Work out the finished part from the listing and answer in its coordinate system (mm). A direction names the side the tool comes from. Give positions to 0.01 mm unless a question says otherwise; leave off trailing zeros. Loops run counter-clockwise (first coordinate to the right, second up) from the corner with the lowest first, then second, coordinate; pieces in that order, holes last. Notation, with made-up numbers: M 48.5,28 L 96.5,28 A14 ccw 96.5,53 Z; hole C 65,21.5 d9. An arc over 180 degrees is marked long. Use a Markdown table: item, result.
```python
from build123d import *

# Parameters (mm, degrees)
SKETCH_W        = 64
SKETCH_H        = 54
PAD_DEPTH       = 17
SKETCH001_W     = 12.371217
SKETCH001_H     = 20
POCKET_DEPTH    = 64.001
SKETCH002_W     = 32
SKETCH002_H     = 23.71851
POCKET001_DEPTH = 34.001
PAD001_DEPTH    = 24
SKETCH005_R     = 10
POCKET002_DEPTH = 64.001
SKETCH006_W     = 20
SKETCH006_H     = 14.23518
POCKET003_DEPTH = 54.001
SKETCH007_R     = 15
POCKET004_DEPTH = 48.001
SKETCH008_R     = 4
POCKET005_DEPTH = 10


with BuildPart() as pocket001:
    # Sketch → Pad (new body, symmetric)
    with BuildSketch(Plane.YZ):
        with Locations((0, 27)):
            Rectangle(SKETCH_W, SKETCH_H)
    extrude(amount=PAD_DEPTH, both=True)

    # Sketch001 → Pocket (cut, through all)
    with BuildSketch(Plane(origin=(0, -32, 0), x_dir=(0, 0, -1), z_dir=(0, -1, 0))):
        with Locations((0.185608, 0)):
            Rectangle(SKETCH001_W, SKETCH001_H)
    extrude(amount=-POCKET_DEPTH, mode=Mode.SUBTRACT)

    # Sketch002 → Pocket001 (cut, through all)
    with BuildSketch(Plane.YZ.offset(17)):
        with Locations((0, 3.140745)):
            Rectangle(SKETCH002_W, SKETCH002_H)
    extrude(amount=-POCKET001_DEPTH, mode=Mode.SUBTRACT)


with BuildPart() as pocket005:
    # Sketch004 → Pad001 (new body, symmetric)
    with BuildSketch(Plane.YZ):
        with BuildLine():
            Line((-16, 0), (-16, 15))
            Line((-16, 15), (16, 15))
            Line((16, 15), (16, 0))
            Line((16, 0), (22, 0))
            Line((22, 0), (22, 38))
            ThreePointArc((22, 38), (0, 60.000055), (-22, 38))
            Line((-22, 0), (-22, 38))
            Line((-16, 0), (-22, 0))
        make_face()
    extrude(amount=PAD001_DEPTH, both=True)

    # Fusion: union Pocket001
    add(pocket001.part)

    # Sketch005 → Pocket002 (cut, through all)
    with BuildSketch(Plane.XZ.offset(32)):
        with Locations((0, 38)):
            Circle(SKETCH005_R)
    extrude(amount=-POCKET002_DEPTH, mode=Mode.SUBTRACT)

    # Sketch006 → Pocket003 (cut, through all)
    with BuildSketch(Plane.XZ.offset(22)):
        with Locations((0, -1.11759)):
            Rectangle(SKETCH006_W, SKETCH006_H)
    extrude(amount=-POCKET003_DEPTH, mode=Mode.SUBTRACT)

    # Sketch007 → Pocket004 (cut, through all)
    with BuildSketch(Plane.YZ.offset(24)):
        with Locations((0, 38)):
            Circle(SKETCH007_R)
    extrude(amount=-POCKET004_DEPTH, mode=Mode.SUBTRACT)

    # Sketch008 → Pocket005 (cut)
    with BuildSketch(Plane.XY.offset(54)):
        with Locations((0, -23.848572)):
            Circle(SKETCH008_R)
        with Locations((0, 24.151428)):
            Circle(SKETCH008_R)
    extrude(amount=-POCKET005_DEPTH, mode=Mode.SUBTRACT)


solid = pocket005.part
```
(1) A cutting plane is placed at D-D (x = 12). Write down the section's boundary in (y, z).
Entries:
| item | result |
|---|---|
| outline | M -32,0 L -16,0 L -16,15 L 16,15 L 16,0 L 32,0 L 32,54 L 15.1,54 A22 ccw -15.1,54 L -32,54 Z; hole C 0,38 d30 |
(2) Consider probe 1 along X at (y, z) = (21, 38); probe 2 along X at (y, z) = (-26.75, 38); probe 3 along Y at (x, z) = (0, 50). Determine where each line is inside the solid, lowest interval first. Write a range as [from, to].
Entries:
| item | result |
|---|---|
| probe 1 | x = [-24, -10], [10, 24] |
| probe 2 | x = [-17, -10], [10, 17] |
| probe 3 | y = [-32, -27.85], [-19.85, -9], [9, 20.15], [28.15, 32] |
(3) Which of the six approach directions +Z, -Z, +X, -X, +Y, -Y give full straight-line access (tool end or side, diameter ignored) to faces 4 (the flat face through (4, -22, 54)), 5 (the flat face through (10, 24, 3)), 6 (the flat face through (-20, 22, 19)), 7 (the flat face through (21, -22, 19)), 8 (the cylindrical face through (-3.996, -23.673, 50.63))?
Entries:
| item | result |
|---|---|
| face 4 | +Z, +X, -X, -Y |
| face 5 | -Z, +Y, -Y |
| face 6 | +Z, -Z, -X, +Y |
| face 7 | +Z, -Z, +X, -Y |
| face 8 | +Z |
(4) A cutting plane is placed at A-A (y = 0). Write down the section's boundary in (x, z).
Entries:
| item | result |
|---|---|
| outline | M -24,15 L 24,15 L 24,23 L -24,23 Z; M -24,53 L 24,53 L 24,60 L -24,60 Z |
(5) Given P1, Ø6.5, axis at y = -26, z = 3, coming from the +X side; P2, Ø2, axis at y = 23.5, z = 49, coming from the -X side; P3, Ø5, axis at x = 0, y = -23.85, coming from the +Z side; P4, Ø24, axis at y = 0, z = 38, coming from the +X side, each flat-ended and moving along its own axis, determine where each tip first touches the part or whether it passes through.
Entries:
| item | result |
|---|---|
| P1 | stops at x = 17 |
| P2 | stops at x = -17 |
| P3 | stops at z = 28.32 |
| P4 | passes through |
(6) A cutting plane is placed at C-C (z = 14). Write down the section's boundary in (x, y).
Entries:
| item | result |
|---|---|
| outline | M -24,-22 L -17,-22 L -17,-32 L 17,-32 L 17,-22 L 24,-22 L 24,-16 L -24,-16 Z; M -24,16 L 24,16 L 24,22 L 17,22 L 17,32 L -17,32 L -17,22 L -24,22 Z |
(7) A cutting plane is placed at B-B (x = 0). Write down the section's boundary in (y, z), and give its area (3 significant figures).
Entries:
| item | result |
|---|---|
| outline | M -32,6 L -16,6 L -16,15 L 16,15 L 16,6 L 32,6 L 32,28 L 11.18,28 A15 cw -11.18,28 L -32,28 Z; M -32,48 L -27.85,48 L -27.85,54 L -32,54 Z; M -19.85,48 L -11.18,48 A15 cw 11.18,48 L 20.15,48 L 20.15,54 L 15.1,54 A22 ccw -15.1,54 L -19.85,54 Z; M 28.15,48 L 32,48 L 32,54 L 28.15,54 Z |
| area | 1,380 mm² |
(8) The mould has two halves that part along Y. Classify faces 1 (the flat face through (-24, -5.2, 23.75)), 2 (the flat face through (0, -16, 7)), 3 (the flat face through (21, 22, 19)): released by +Y, released by -Y, zero draft, split by the parting line, or undercut.
Entries:
| item | result |
|---|---|
| face 1 | zero draft |
| face 2 | undercut |
| face 3 | released by +Y |
